For this review, take the finished solid that the model builds, in its own axes (mm). Face numbers are marked on the shaded views. A direction names the side the tool comes from. Coordinates: 2 decimals unless noted, no trailing zeros. Write each loop counter-clockwise with the first axis right and the second up, starting at its lowest first coordinate (ties: lowest second). Pieces come first, ordered by that corner, then holes.
```python
from build123d import *

# Parameters (mm, degrees)
SKETCH1_W                        = 25.4
SKETCH1_H                        = 25.4
BOSS_EXTRUDE1_DEPTH              = 6.35
SKETCH2_W                        = 25.4
SKETCH2_H                        = 31.75
BOSS_EXTRUDE2_DEPTH              = 6.35
FILLET1_R                        = 2.54
F_11_64_0_17188_DIAMETER_HOLE1_D = 4.365752
F_11_64_0_17188_DIAMETER_HOLE2_D = 4.365752


with BuildPart() as part:
    # Sketch1 → Boss-Extrude1 (new body)
    with BuildSketch(Plane(origin=(0, 0, 0), x_dir=(1, 0, 0), z_dir=(0, 1, 0))):
        Rectangle(SKETCH1_W, SKETCH1_H)
    extrude(amount=BOSS_EXTRUDE1_DEPTH)

    # Sketch2 → Boss-Extrude2 (add)
    with BuildSketch(Plane(origin=(0, 0, -12.7), x_dir=(-1, 0, 0), z_dir=(0, 0, -1))):
        with Locations((0, 15.875)):
            Rectangle(SKETCH2_W, SKETCH2_H)
    extrude(amount=BOSS_EXTRUDE2_DEPTH)

    # Fillet1
    fillet1_edges = [part.edges().sort_by_distance(p)[0] for p in [
        (0, 31.75, -12.7),
        (-12.7, 31.75, -15.875),
        (12.7, 31.75, -15.875),
        (0, 6.35, 12.7),
        (0, 31.75, -19.05),
        (0, 0, 12.7),
        (12.7, 3.175, 12.7),
        (-12.7, 3.175, 12.7),
        (0, 6.35, -12.7),
    ]]
    fillet(fillet1_edges, radius=FILLET1_R)

    # 11/64 (0.17188) Diameter Hole1 (through all)
    with Locations(Plane(origin=(0, 6.35, 0), x_dir=(1, 0, 0), z_dir=(0, 1, 0))):
        with Locations((-6.35, 0), (6.35, 0)):
            Hole(F_11_64_0_17188_DIAMETER_HOLE1_D / 2)

    # 11/64 (0.17188) Diameter Hole2 (through all)
    with Locations(Plane.XY.offset(-12.7)):
        with Locations((6.35, 19.05), (-6.35, 19.05)):
            Hole(F_11_64_0_17188_DIAMETER_HOLE2_D / 2)


solid = part.part
```
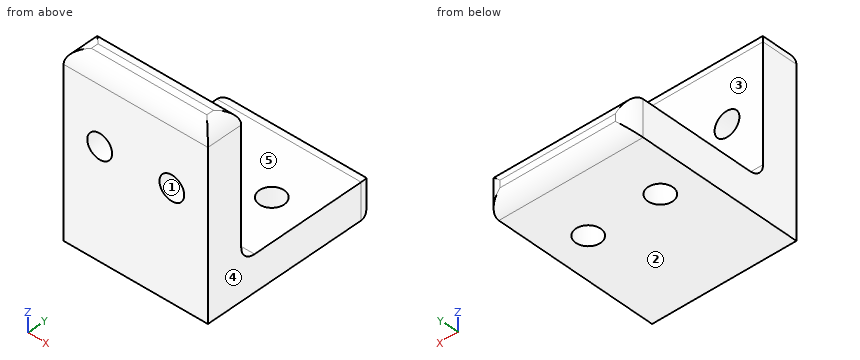
Q1. Draft analysis for pull direction Z (two halves, no side actions). For the marked faces 1, 2 and 3, state which applies: +Z half, -Z half, draft (parallel to the pull), parting line (faces both ways), or undercut.
Ans:
face 1: undercut
face 2: -Z half
face 3: draft
Q2. Clearance check with flat-ended pins moving along their axes: pin 1 Ø1.5 at (x, y) = (-7, 21.5) entering from +Z; pin 2 Ø2 at (x, y) = (3, 9) entering from +Z; pin 3 Ø3 at (x, y) = (-5, 6.5) entering from +Z. State where each tip first meets the part, or that it passes through.
Ans:
pin 1: stops at z = -12.7
pin 2: stops at z = -12.54
pin 3: stops at z = 12.4
Q3. For probe 1 along Y at (x, z) = (6.35, -16); probe 2 along X at (y, z) = (19, -16); probe 3 along Z at (x, y) = (6.35, 3.75), list the stretches that pass through material, from the lowest coordinate up.
Ans:
probe 1: y = 0 to 16.87, 21.23 to 31.75
probe 2: x = -12.7 to -8.53, -4.17 to 4.17, 8.53 to 12.7
probe 3: z = -19.05 to -2.18, 2.18 to 12.7
Q4. Add section D-D (x = -0.25). State the section outline as (y, z) points.
Ans:
outline: (0, -19.05) - (29.21, -19.05) arc R2.54 ccw to (31.75, -16.51) - (31.75, -15.24) arc R2.54 ccw to (29.21, -12.7) - (8.89, -12.7) arc R2.54 cw to (6.35, -10.16) - (6.35, 10.16) arc R2.54 ccw to (3.81, 12.7) - (2.54, 12.7) arc R2.54 ccw to (0, 10.16) - close
Q5. Add section B-B (x = 6.35). State the section outline as (y, z) points, then the cut area to 3 significant figures.
Ans:
outline: (0, -19.05) - (16.87, -19.05) - (16.87, -12.7) - (8.89, -12.7) arc R2.54 cw to (6.35, -10.16) - (6.35, -2.18) - (0, -2.18) - close; (0, 2.18) - (6.35, 2.18) - (6.35, 10.16) arc R2.54 ccw to (3.81, 12.7) - (2.54, 12.7) arc R2.54 ccw to (0, 10.16) - close; (21.23, -19.05) - (29.21, -19.05) arc R2.54 ccw to (31.75, -16.51) - (31.75, -15.24) arc R2.54 ccw to (29.21, -12.7) - (21.23, -12.7) - close
area: 303 mm2
Q6. Tool access review of the marked faces 4 and 5: name each direction out of +Z, -Z, +X, -X, +Y, -Y from which nothing blocks a thin tool from reaching the whole face with its end or side.
Ans:
face 4: +Z, -Z, +X, +Y, -Y
face 5: +Z, +X, -X, +Y
Q7. Add section C-C (y = 19.05). State the section outline as (x, z) points, then the cut area to 3 significant figures.
Ans:
outline: (-12.7, -19.05) - (-8.53, -19.05) - (-8.53, -12.7) - (-12.7, -12.7) - close; (-4.17, -19.05) - (4.17, -19.05) - (4.17, -12.7) - (-4.17, -12.7) - close; (8.53, -19.05) - (12.7, -19.05) - (12.7, -12.7) - (8.53, -12.7) - close
area: 106 mm2
Q8. Add section A-A (z = 0). State the section outline as (x, y) points.
Ans:
outline: (-12.7, 0) - (-8.53, 0) - (-8.53, 6.35) - (-12.7, 6.35) - close; (-4.17, 0) - (4.17, 0) - (4.17, 6.35) - (-4.17, 6.35) - close; (8.53, 0) - (12.7, 0) - (12.7, 6.35) - (8.53, 6.35) - close
